from build123d import *

# Parameters (mm, degrees)
PRISM001_DEPTH = 15
PRISM_DEPTH    = 15


with BuildPart() as prism001:
    # Prism001 → Prism001 (new body)
    with BuildSketch(Plane.XY):
        Polygon((88, 0), (-44, 76.210236), (-44, -76.210236), align=None)
    extrude(amount=PRISM001_DEPTH)


with BuildPart() as cut:
    # Prism → Prism (new body)
    with BuildSketch(Plane.XY):
        Polygon((138, 0), (-69, 119.511506), (-69, -119.511506), align=None)
    extrude(amount=PRISM_DEPTH)

    # Cut: cut Prism001
    add(prism001.part, mode=Mode.SUBTRACT)


solid = cut.part
Input: part model. Units: mm. Frame: model coordinates. A direction names the side the tool comes from. Give positions to 0.01 mm unless a question says otherwise; leave off trailing zeros. Order: outer loops, then holes, each group sorted by start corner. A loop starts at its lowest first (then second) coordinate and runs counter-clockwise, first axis right, second up.
Q1. Draft query along Y for faces 3 (the flat face through (34, -35, 0)), 4 (the flat face through (22.924, 37.572, 7.395)), 5 (the flat face through (35.95, 58.92, 7.4)), 6 (the flat face through (21.076, -38.639, 7.395)). Return one class per face: +Y half, -Y half, draft (parallel to the pull), parting line (faces both ways), or undercut.
Checked values:
face 3: draft
face 4: undercut
face 5: +Y half
face 6: undercut
Q2. Set-up query: faces 1 (the flat face through (-44, 1, 7)), 2 (the flat face through (-69, 2, 7)). Return all of +Z, -Z, +X, -X, +Y, -Y with unobstructed straight access to the full face (end or side cutting, diameter ignored); none if empty.
Checked values:
face 1: +Z, -Z
face 2: +Z, -Z, -X, +Y, -Y
Q3. Contact query for flat-ended pins moving along their axis: pin 1 Ø4.5 at (y, z) = (16, 4.5) entering from +X; pin 2 Ø6 at (y, z) = (-5.5, 13) entering from +X; pin 3 Ø4 at (x, z) = (-25, 8) entering from -Y. Output: stop coordinate, or through.
Checked values:
pin 1: stops at x = 114.18
pin 2: stops at x = 133.67
pin 3: stops at y = -95.26
Q4. Ray query, probe 1 along X at (y, z) = (-61, 10.75); probe 2 along Y at (x, z) = (21.5, 11.25); probe 3 along X at (y, z) = (73.5, 8.75). Return the intervals inside material, ascending.
Checked values:
probe 1: x = -69 to -44, -17.66 to 32.34
probe 2: y = -67.26 to -38.39, 38.39 to 67.26
probe 3: x = -69 to -44, -39.31 to 10.69
Q5. Section A-A on x = 27. Output: boundary loops of the cut face in (y, z), and give its area (3 significant figures).
Checked values:
outline: (-64.09, 0) - (-35.22, 0) - (-35.22, 15) - (-64.09, 15) - close; (35.22, 0) - (64.09, 0) - (64.09, 15) - (35.22, 15) - close
area: 866 mm2
Q6. Section B-B on z = 6.25. Output: boundary loops of the cut face in (x, y).
Checked values:
outline: (-69, -119.51) - (138, 0) - (-69, 119.51) - close; hole (-44, -76.21) - (88, 0) - (-44, 76.21) - close
Q7. Section C-C on y = -63. Output: boundary loops of the cut face in (x, z), and give its area (4 significant figures).
Checked values:
outline: (-69, 0) - (-44, 0) - (-44, 15) - (-69, 15) - close; (-21.12, 0) - (28.88, 0) - (28.88, 15) - (-21.12, 15) - close
area: 1,125 mm2
Q8. Section D-D on y = 104. Output: boundary loops of the cut face in (x, z).
Checked values:
outline: (-69, 0) - (-42.13, 0) - (-42.13, 15) - (-69, 15) - close
